Autodesk Inventor part; units mm, degrees
ref_plane "YZ Plane" through (0, 0, 0) normal (1, 0, 0) x (0, 1, 0)
ref_plane "XZ Plane" through (0, 0, 0) normal (0, 1, 0) x (-1, 0, 0)
ref_plane "XY Plane" through (0, 0, 0) normal (0, 0, 1) x (1, 0, 0)
sketch "Sketch1" plane through (0, 0, 0) normal (0, 0, 1) x (1, 0, 0)
  line L0 (-12.7, -12.7) -> (12.7, -12.7)
  line L1 (12.7, -12.7) -> (12.7, 12.7)
  line L2 (12.7, 12.7) -> (-12.7, 12.7)
  line L3 (-12.7, 12.7) -> (-12.7, -12.7)
  line L4 (-12.7, -12.7) -> (12.7, 12.7) construction
  line L5 (12.7, -12.7) -> (-12.7, 12.7) construction
  line L6 (-10.16, 10.16) -> (10.16, 10.16)
  line L7 (10.16, 10.16) -> (10.16, -10.16)
  line L8 (10.16, -10.16) -> (-10.16, -10.16)
  line L9 (-10.16, -10.16) -> (-10.16, 10.16)
  point P0 (0, 0)
  dimension "l1" = 25.4
  dimension "l2" = 25.4
  dimension "wt" = 2.54
extrude "Extrusion1" add sketch "Sketch1" against normal blind 914.4
sketch "Sketch2" plane through (-12.7, 12.7, 0) normal (0, 1, 0) x (1, 0, 0)
  line L0 (25.4, 0) -> (0, 0)
  line L1 (25.4, 0) -> (25.4, 914.4)
  line L2 (0, 914.4) -> (25.4, 914.4)
  line L3 (0, 0) -> (0, 914.4)
  point P0 (12.7, 0)
  point P1 (12.7, 12.7)
  dimension "d5" = 25.4
  dimension "d6" = 12.7
  dimension "d7" = 12.7
hole "Hole3" at (0, 12.7, -12.7) direction (0, -1, 0) diameter 4.0894 end through all
sketch "Sketch3" plane through (12.7, -12.7, 0) normal (1, 0, 0) x (0, 0, -1)
  line L0 (0, 0) -> (0, 25.4)
  line L1 (0, 0) -> (914.4, 0)
  line L2 (914.4, 25.4) -> (914.4, 0)
  line L3 (0, 25.4) -> (914.4, 25.4)
  point P0 (0, 12.7)
  point P1 (25.4, 12.7)
  dimension "d22" = 25.4
  dimension "d23" = 12.7
  dimension "d24" = 25.4
hole "Hole4" [suppressed]
pattern_linear "Rectangular Pattern1" count 37 spacing 25.4 along (0, 0, -1) of "Hole3"
pattern_linear "Rectangular Pattern2" [suppressed]
properties part number "versatubing long boy" material "Aluminum 6061"
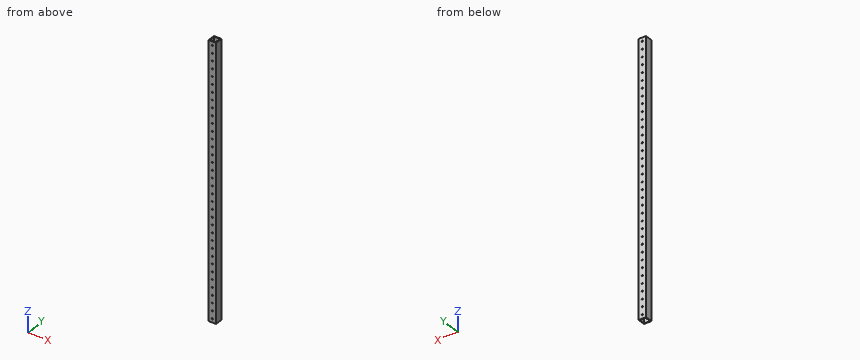
Here's how the part is built. I have some questions about the finished solid (model axes, mm). Coordinates: 2 decimals unless noted, no trailing zeros. Order: outer loops, then holes, each group sorted by start corner. A loop starts at its lowest first (then second) coordinate and runs counter-clockwise, first axis right, second up.
Item 1: I need wall thicknesses on line 1 (X direction, y = 4.5, z = -544.5); line 2 (X direction, y = -11, z = -901.7). Which ranges of each line are inside material? Lowest first, please.
Result sheet:
line 1: x = -12.7 to -10.16, 10.16 to 12.7
line 2: x = -12.7 to -2.04, 2.04 to 12.7
Item 2: If we section it at B-B on z = -610.5: List the corners of the cut face in (x, y) for me.
Result sheet:
outline: (-12.7, -12.7) - (12.7, -12.7) - (12.7, 12.7) - (-12.7, 12.7) - close; hole (-10.16, -10.16) - (10.16, -10.16) - (10.16, 10.16) - (-10.16, 10.16) - close
Item 3: For P1, Ø6.5, axis at x = 0, z = -342.9, coming from the -Y side; P2, Ø2.5, axis at x = 0, z = -571.5, coming from the -Y side, each with a flat end and sliding along its axis, tell me the tip position at first contact or that it passes through.
Result sheet:
P1: stops at y = -12.7
P2: passes through
Item 4: If we section it at A-A on y = 3: List the corners of the cut face in (x, z) for me.
Result sheet:
outline: (-12.7, -914.4) - (-10.16, -914.4) - (-10.16, 0) - (-12.7, 0) - close; (10.16, -914.4) - (12.7, -914.4) - (12.7, 0) - (10.16, 0) - close
